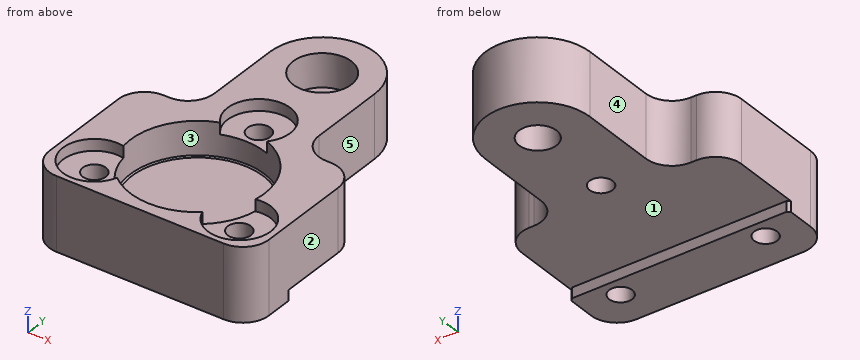
from build123d import *

# Parameters (mm, degrees)
BOSS_EXTRUDE1_DEPTH                              = 14
SKETCH2_R                                        = 12.8
CUT_EXTRUDE1_DEPTH                               = 6.608
CBORE_FOR_1_4_SOCKET_HEAD_CAP_SCREW1_D           = 7.14248
CBORE_FOR_1_4_SOCKET_HEAD_CAP_SCREW1_CBORE_D     = 11.1125
CBORE_FOR_1_4_SOCKET_HEAD_CAP_SCREW1_CBORE_DEPTH = 6.35
SKETCH5_R                                        = 6
CUT_EXTRUDE2_DEPTH                               = 2.2
CIRPATTERN2_COUNT                                = 3
TAPPED_HOLE_FOR_8_32_HELICOIL1_D                 = 4.3942
TAPPED_HOLE_FOR_8_32_HELICOIL1_DEPTH             = 13.322
TAPPED_HOLE_FOR_8_32_HELICOIL1_TIP               = 1.320150866
SKETCH8_W                                        = 42
SKETCH8_H                                        = 46.9
CUT_EXTRUDE3_DEPTH                               = 2
CHAMFER1_SIZE                                    = 0.508
CHAMFER2_SIZE                                    = 0.254


with BuildPart() as part:
    # Sketch1 → Boss-Extrude1 (new body)
    with BuildSketch(Plane.XY):
        with BuildLine():
            Line((-10, 18), (-10, 32.5))
            ThreePointArc((-10, 32.5), (0, 42.5), (10, 32.5))
            Line((10, 32.5), (10, 18))
            ThreePointArc((10, 18), (11.464466094, 14.464466094), (15, 13))
            Line((15, 13), (16, 13))
            ThreePointArc((16, 13), (19.535533906, 11.535533906), (21, 8))
            Line((21, 8), (21, -10))
            ThreePointArc((21, -10), (19.535533906, -13.535533906), (16, -15))
            Line((16, -15), (-16, -15))
            ThreePointArc((-16, -15), (-19.535533906, -13.535533906), (-21, -10))
            Line((-21, -10), (-21, 8))
            ThreePointArc((-21, 8), (-19.535533906, 11.535533906), (-16, 13))
            Line((-16, 13), (-15, 13))
            ThreePointArc((-15, 13), (-11.464466094, 14.464466094), (-10, 18))
        make_face()
    extrude(amount=BOSS_EXTRUDE1_DEPTH)

    # Sketch2 → Cut-Extrude1 (cut)
    with BuildSketch(Plane.XY.offset(14)):
        Circle(SKETCH2_R)
    extrude(amount=-CUT_EXTRUDE1_DEPTH, mode=Mode.SUBTRACT)

    # CBORE for 1_4 Socket Head Cap Screw1 (through all)
    with Locations(Plane.XY.offset(14)):
        with Locations((0, 32.5)):
            CounterBoreHole(CBORE_FOR_1_4_SOCKET_HEAD_CAP_SCREW1_D / 2, CBORE_FOR_1_4_SOCKET_HEAD_CAP_SCREW1_CBORE_D / 2, CBORE_FOR_1_4_SOCKET_HEAD_CAP_SCREW1_CBORE_DEPTH)

    # Sketch5 → Cut-Extrude2 (cut)
    with BuildSketch(Plane.XY.offset(14)):
        with Locations((0, 16)):
            Circle(SKETCH5_R)
    cut_extrude2 = extrude(amount=-CUT_EXTRUDE2_DEPTH, mode=Mode.SUBTRACT)

    # CirPattern2: Cut-Extrude2 ×3 about axis
    cirpattern2_axis = Axis((0, 0, 0), (0, 0, 1))
    for i in range(1, CIRPATTERN2_COUNT):
        add(cut_extrude2.rotate(cirpattern2_axis, i * 360 / CIRPATTERN2_COUNT), mode=Mode.SUBTRACT)

    # Tapped Hole for _8-32 Helicoil1
    with Locations(Plane.XY.offset(11.8)):
        with Locations((0, 16), (-13.856406461, -8), (13.856406461, -8)):
            Hole(TAPPED_HOLE_FOR_8_32_HELICOIL1_D / 2, depth=TAPPED_HOLE_FOR_8_32_HELICOIL1_DEPTH)
            with Locations((0, 0, -(TAPPED_HOLE_FOR_8_32_HELICOIL1_DEPTH + TAPPED_HOLE_FOR_8_32_HELICOIL1_TIP / 2))):  # 118° drill point
                Cone(0, TAPPED_HOLE_FOR_8_32_HELICOIL1_D / 2, TAPPED_HOLE_FOR_8_32_HELICOIL1_TIP, mode=Mode.SUBTRACT)

    # Sketch8 → Cut-Extrude3 (cut)
    with BuildSketch(Plane(origin=(0, 0, 0), x_dir=(-1, 0, 0), z_dir=(0, 0, -1))):
        with Locations((0, 19.05)):
            Rectangle(SKETCH8_W, SKETCH8_H)
    extrude(amount=-CUT_EXTRUDE3_DEPTH, mode=Mode.SUBTRACT)

    # Chamfer1
    chamfer1_edges = [part.edges().sort_by_distance(p)[0] for p in [
        (21, -4.4, 1),
        (-21, -4.4, 1),
    ]]
    chamfer(chamfer1_edges, length=CHAMFER1_SIZE)

    # Chamfer2
    chamfer2_edges = [part.edges().sort_by_distance(p)[0] for p in [
        (-12.8, 0, 7.392),
    ]]
    chamfer(chamfer2_edges, length=CHAMFER2_SIZE)


solid = part.part
Part model, mm, in its own coordinate system. Face numbers are marked on the shaded views. A direction names the side the tool comes from. Coordinates: 2 decimals unless noted, no trailing zeros. Loops run counter-clockwise (first coordinate to the right, second up) from the corner with the lowest first, then second, coordinate; pieces in that order, holes last. Notation, with made-up numbers: M 68.5,14.25 L 78.5,14.25 A28 ccw 78.5,41.25 Z; hole C -19.75,80.25 d9. An arc over 180 degrees is marked long. Use a Markdown table: item, result. Add a question column.
Q1. Cut at B-B (z = 9.25). Write the cut outline in (x, y).
Q2. Cut at D-D (z = 5.25). Write the cut outline in (x, y), and give its area (3 significant figures).
Q3. Pin check, flat tips, straight feed: P1, Ø6, axis at y = 22.5, z = 3, coming from the -X side; P2, Ø14.5, axis at x = 0, y = 32.5, coming from the -Z side; P3, Ø4, axis at y = 16, z = 6, coming from the -X side. Stop position of each tip, or through.
Q4. Cut at A-A (x = 0). Write the cut outline in (y, z), and give its area (3 significant figures).
Q5. Which spindle directions (+Z, -Z, +X, -X, +Y, -Y) get a long thin tool onto all of the face, cutting with end or side? Do the marked faces 1, 2, 3, 4 and 5. Say none if no direction does.
Q6. Cut at C-C (y = 0). Write the cut outline in (x, z), and give its area (3 significant figures).
Q7. Probe L1, parallel to Y at x = 0, z = 10; L2, parallel to Y at x = 0, z = 6.25; L3, parallel to X at y = -8, z = 13.25. List the from-to ranges inside material, lowest first.
Worked out:
| question | item | result |
|---|---|---|
| 1 | outline | M -21,-10 A5 ccw -16,-15 L 16,-15 A5 ccw 21,-10 L 21,8 A5 ccw 16,13 L 15,13 A5 cw 10,18 L 10,32.5 A10 ccw -10,32.5 L -10,18 A5 cw -15,13 L -16,13 A5 ccw -21,8 Z; hole C -13.86,-8 d4.39; hole C 0,0 d25.6; hole C 0,32.5 d11.11; hole C 0,16 d4.39; hole C 13.86,-8 d4.39 |
| 2 | outline | M -21,-10 A5 ccw -16,-15 L 16,-15 A5 ccw 21,-10 L 21,8 A5 ccw 16,13 L 15,13 A5 cw 10,18 L 10,32.5 A10 ccw -10,32.5 L -10,18 A5 cw -15,13 L -16,13 A5 ccw -21,8 Z; hole C -13.86,-8 d4.39; hole C 0,32.5 d7.14; hole C 0,16 d4.39; hole C 13.86,-8 d4.39 |
| 2 | area | 1,630 mm2 |
| 3 | P1 | stops at x = -10 |
| 3 | P2 | stops at z = 2 |
| 3 | P3 | stops at x = -12 |
| 4 | outline | M -15,0 L -4.4,0 L -4.4,2 L 13.8,2 L 13.8,11.8 L 12.8,11.8 L 12.8,7.65 L 12.55,7.39 L -12.55,7.39 L -12.8,7.65 L -12.8,14 L -15,14 Z; M 18.2,2 L 28.93,2 L 28.93,7.65 L 26.94,7.65 L 26.94,14 L 22,14 L 22,11.8 L 18.2,11.8 Z; M 36.07,2 L 42.5,2 L 42.5,14 L 38.06,14 L 38.06,7.65 L 36.07,7.65 Z |
| 4 | area | 368 mm2 |
| 5 | face 1 | -Z, +X, -X, +Y |
| 5 | face 2 | +Z, -Z, +X, +Y, -Y |
| 5 | face 3 | +Z |
| 5 | face 4 | +Z, -Z, -X, +Y |
| 5 | face 5 | +Z, -Z, +X, +Y |
| 6 | outline | M -21,2 L 21,2 L 21,14 L 12.8,14 L 12.8,7.65 L 12.55,7.39 L -12.55,7.39 L -12.8,7.65 L -12.8,14 L -21,14 Z |
| 6 | area | 335 mm2 |
| 7 | L1 | y = -15 to -12.8, 12.8 to 13.8, 18.2 to 26.94, 38.06 to 42.5 |
| 7 | L2 | y = -15 to 13.8, 18.2 to 28.93, 36.07 to 42.5 |
| 7 | L3 | x = -21 to -19.86, 19.86 to 21 |
